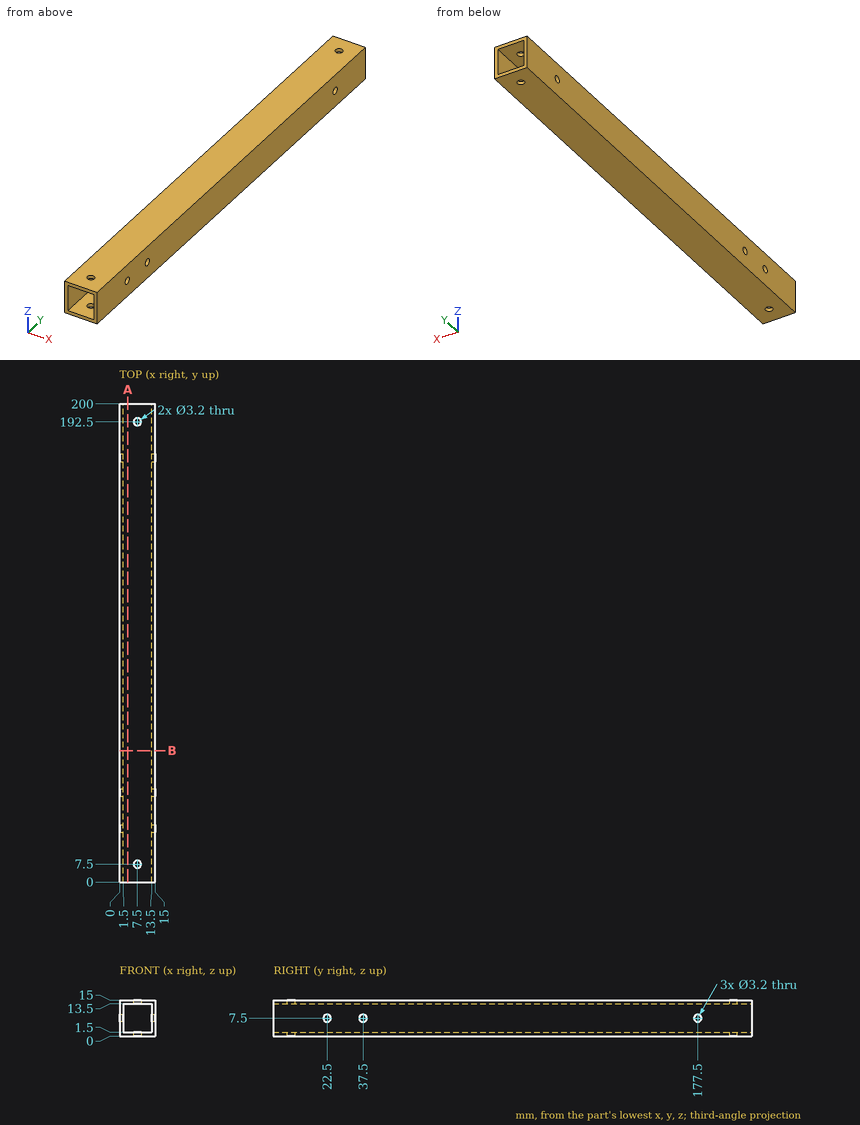
Here's the drawing with two shaded views (mm, measured from the low corner). I have some questions. Coordinates: 2 decimals unless noted, no trailing zeros. Order: outer loops, then holes, each group sorted by start corner. A loop starts at its lowest first (then second) coordinate and runs counter-clockwise, first axis right, second up.
Item 1: I need wall thicknesses on line 1 (Y direction, x = 0.5, z = 7.5); line 2 (X direction, y = 192.5, z = 0.3); line 3 (X direction, y = 190, z = 2). Which ranges of each line are inside material? Lowest first, please.
Result sheet:
line 1: y = 0 to 20.9, 24.1 to 35.9, 39.1 to 175.9, 179.1 to 200
line 2: x = 0 to 5.9, 9.1 to 15
line 3: x = 0 to 1.5, 13.5 to 15
Item 2: If we section it at A-A on x = 3.5: List the corners of the cut face in (y, z) for me.
Result sheet:
outline: (0, 0) - (200, 0) - (200, 1.5) - (0, 1.5) - close; (0, 13.5) - (200, 13.5) - (200, 15) - (0, 15) - close
Item 3: For P1, Ø2.5, axis at x = 7.5, y = 7.5, coming from the -Z side, with a flat end and sliding along its axis, tell me the tip position at first contact or that it passes through.
Result sheet:
P1: passes through
Item 4: If we section it at B-B on y = 55: List the corners of the cut face in (x, z) for me.
Result sheet:
outline: (0, 0) - (15, 0) - (15, 15) - (0, 15) - close; hole (1.5, 1.5) - (13.5, 1.5) - (13.5, 13.5) - (1.5, 13.5) - close
